The model under review builds one solid part; all positions refer to its coordinate system, in mm. A direction names the side the tool comes from. Coordinates: 2 decimals unless noted, no trailing zeros. Write each loop counter-clockwise with the first axis right and the second up, starting at its lowest first coordinate (ties: lowest second). Pieces come first, ordered by that corner, then holes.
1) For line 1 (Y direction, x = -0.55, z = 2.9); line 2 (Y direction, x = 3.7, z = 2.6); line 3 (X direction, y = -3.3, z = 0.45), list the stretches that pass through material, from the lowest coordinate up.
2) Mouldability with a two-part tool opening along Y and no side actions: class faces 3 (the flat face through (2, -4.483, 2)), 4 (the flat face through (-1, -0.165, 2)), 5 (the flat face through (1, -4.737, 2)) as released by +Y, released by -Y, zero draft, split by the parting line, or undercut.
3) Add section C-C, the plane x = 2.3. State the section outline as (y, z) points.
4) For P1, Ø1.5, axis at y = -1.5, z = 1.5, coming from the +X side; P2, Ø1, axis at x = 3, z = 2, coming from the +Y side; P3, Ø2, axis at x = 0.5, y = -2.5, coming from the -Z side, all flat-tipped, find the tip position at first contact; note any pin that passes through.
5) Machinability: for faces 1 (the flat face through (-1, -0.419, 2)), 2 (the flat face through (-1.595, -2, 2)), which of the approach directions +Z, -Z, +X, -X, +Y, -Y give a long, thin tool a straight path to every point of the face, cutting with its end or side? Answer none if there is none.
6) Add section A-A, the plane z = 2.65. State the section outline as (x, y) points.
7) Add section B-B, the plane y = -2.9. State the section outline as (x, z) points, then the cut area to 3 significant figures.
Autodesk Inventor part; units mm, degrees
ref_plane "YZ Plane" through (0, 0, 0) normal (1, 0, 0) x (0, 1, 0)
ref_plane "XZ Plane" through (0, 0, 0) normal (0, 1, 0) x (-1, 0, 0)
ref_plane "XY Plane" through (0, 0, 0) normal (0, 0, 1) x (1, 0, 0)
sketch "Sketch1" plane through (0, 0, 0) normal (0, 0, 1) x (1, 0, 0)
  line L0 (-1.3413, -0.4194) -> (0, -0.4194)
  line L1 (-1.3413, -4.7374) -> (-1.3413, -0.4194)
  line L2 (0, -0.1654) -> (-1.5953, -0.1654)
  line L3 (-1.5953, -0.1654) -> (-1.5953, -4.7374)
  line L4 (-1.3413, -4.7374) -> (-1.5953, -4.7374)
  line L5 (0, -0.4194) -> (0, -0.1654)
  point P0 (0, 0)
  dimension "d1" = 0.254
  dimension "d8" = 4.572
extrude "Extrusion1" add sketch "Sketch1" along normal blind 3.048
sketch "Sketch2" plane through (0, 0, 3.048) normal (0, 0, 1) x (1, 0, 0)
  line L0 (-1.3413, -4.7374) -> (4.2975, -4.7374)
  line L1 (4.2975, -4.7374) -> (4.2975, -4.4834)
  line L2 (4.2975, -4.4834) -> (-1.3413, -4.4834)
  line L3 (-1.3413, -4.4834) -> (-1.3413, -4.7374)
  dimension "d4" = 5.6388
  dimension "d5" = 0.254
extrude "Extrusion2" add sketch "Sketch2" against normal up to surface (3.048 mm away)
Geometry results:
1. line 1: y = -4.74 to -4.48, -0.42 to -0.17
1. line 2: y = -4.74 to -4.48
1. line 3: x = -1.6 to -1.34
2. face 3: undercut
2. face 4: released by +Y
2. face 5: released by -Y
3. outline: (-4.74, 0) - (-4.48, 0) - (-4.48, 3.05) - (-4.74, 3.05) - close
4. P1: stops at x = -1.34
4. P2: stops at y = -4.48
4. P3: passes through
5. face 1: +Z, -Z, +X
5. face 2: +Z, -Z, -X, +Y, -Y
6. outline: (-1.6, -4.74) - (4.3, -4.74) - (4.3, -4.48) - (-1.34, -4.48) - (-1.34, -0.42) - (0, -0.42) - (0, -0.17) - (-1.6, -0.17) - close
7. outline: (-1.6, 0) - (-1.34, 0) - (-1.34, 3.05) - (-1.6, 3.05) - close
7. area: 0.774 mm2
